from build123d import *

# Parameters (mm, degrees)
SKETCH_W      = 42
SKETCH_H      = 42
PAD_DEPTH     = 40
CHAMFER_SIZE  = 4
SKETCH001_W   = 44
SKETCH001_H   = 44
POCKET_DEPTH  = 32
PAD001_DEPTH  = 8
SKETCH003_R   = 11
SKETCH003_R_2 = 4.75
PAD002_DEPTH  = 2
PAD003_DEPTH  = 24.5
SKETCH005_R   = 1.7
HOLE_DEPTH    = 4.5
HOLE_TIPS_R   = 1.7


with BuildPart() as part:
    # Sketch → Pad (new body)
    with BuildSketch(Plane.XY):
        Rectangle(SKETCH_W, SKETCH_H)
    extrude(amount=PAD_DEPTH)

    # Chamfer
    chamfer_edges = [part.edges().sort_by_distance(p)[0] for p in [
        (21, -21, 20),
        (-21, -21, 20),
        (21, 21, 20),
        (-21, 21, 20),
    ]]
    chamfer(chamfer_edges, length=CHAMFER_SIZE)

    # Sketch001 (on Face5 of Chamfer) → Pocket (cut)
    with BuildSketch(Plane.XY.offset(40)):
        Rectangle(SKETCH001_W, SKETCH001_H)
        Polygon((-21, -12.868272), (-12.868272, -21), (12.868272, -21), (21, -12.868272), (21, 12.868272), (12.868272, 21), (-12.868272, 21), (-21, 12.868272), align=None, mode=Mode.SUBTRACT)
    extrude(amount=-POCKET_DEPTH, mode=Mode.SUBTRACT)

    # Sketch002 (on Face9 of Pocket) → Pad001 (join)
    with BuildSketch(Plane.XY.offset(40)):
        Polygon((-17, 21), (17, 21), (21, 17), (21, -17), (17, -21), (-17, -21), (-21, -17), (-21, 17), align=None)
    extrude(amount=-PAD001_DEPTH)

    # Sketch003 (on Face26 of Pad001) → Pad002 (join)
    with BuildSketch(Plane.XY.offset(40)):
        Circle(SKETCH003_R)
        Circle(SKETCH003_R_2, mode=Mode.SUBTRACT)
    extrude(amount=PAD002_DEPTH)

    # Sketch004 (on Face14 of Pad002) → Pad003 (join)
    with BuildSketch(Plane.XY.offset(40)):
        with BuildLine():
            ThreePointArc((-2, -1.5), (2.5, 0), (-2, 1.5))
            Line((-2, 1.5), (-2, -1.5))
        make_face()
    extrude(amount=PAD003_DEPTH)

    # Sketch005 (on Face14 of Pad003) → Hole (cut)
    with BuildSketch(Plane.XY.offset(40)):
        with Locations((-15.5, 15.5)):
            Circle(SKETCH005_R)
        with Locations((15.5, 15.5)):
            Circle(SKETCH005_R)
        with Locations((15.5, -15.5)):
            Circle(SKETCH005_R)
        with Locations((-15.5, -15.5)):
            Circle(SKETCH005_R)
    extrude(amount=-HOLE_DEPTH, mode=Mode.SUBTRACT)

    # Hole tips → Hole tip 1 section 0
    with BuildSketch(Plane.XY.offset(35.5), mode=Mode.PRIVATE) as hole_tip_1_s0:
        with Locations((-15.5, 15.5)):
            Circle(HOLE_TIPS_R)
    loft([hole_tip_1_s0.sketch, Vertex(-15.5, 15.5, 34.478537)], mode=Mode.SUBTRACT)

    # Hole tips → Hole tip 2 section 0
    with BuildSketch(Plane.XY.offset(35.5), mode=Mode.PRIVATE) as hole_tip_2_s0:
        with Locations((15.5, 15.5)):
            Circle(HOLE_TIPS_R)
    loft([hole_tip_2_s0.sketch, Vertex(15.5, 15.5, 34.478537)], mode=Mode.SUBTRACT)

    # Hole tips → Hole tip 3 section 0
    with BuildSketch(Plane.XY.offset(35.5), mode=Mode.PRIVATE) as hole_tip_3_s0:
        with Locations((15.5, -15.5)):
            Circle(HOLE_TIPS_R)
    loft([hole_tip_3_s0.sketch, Vertex(15.5, -15.5, 34.478537)], mode=Mode.SUBTRACT)

    # Hole tips → Hole tip 4 section 0
    with BuildSketch(Plane.XY.offset(35.5), mode=Mode.PRIVATE) as hole_tip_4_s0:
        with Locations((-15.5, -15.5)):
            Circle(HOLE_TIPS_R)
    loft([hole_tip_4_s0.sketch, Vertex(-15.5, -15.5, 34.478537)], mode=Mode.SUBTRACT)


solid = part.part
Check sheet for the modelled part. Datum: model origin and axes. Units: mm. A direction names the side the tool comes from. Coordinates: 2 decimals unless noted, no trailing zeros. Loops run counter-clockwise (first coordinate to the right, second up) from the corner with the lowest first, then second, coordinate; pieces in that order, holes last. Notation, with made-up numbers: (45, -20) -> (87, -20) arc R21 ccw to (87, 11) -> close; hole circle Ø4 at (-14, 81.25). An arc over 180 degrees is marked (long way). Answer in a Markdown table with one row per item.
1. Sectioned sample at D-D, the plane z = 19.5. Record the boundary of the cut face in (x, y).
Check values:
| item | result |
|---|---|
| outline | (-21, -12.87) -> (-12.87, -21) -> (12.87, -21) -> (21, -12.87) -> (21, 12.87) -> (12.87, 21) -> (-12.87, 21) -> (-21, 12.87) -> close |
2. Release check for a two-part mould opening along X. For faces 1 (the face through (17.07, -16.15, 37.78)), 2 (the face through (16.88, -16.99, 20.17)), 3 (the face through (-2.38, -10.74, 40.99)), 4 (the face through (-19, -19, 4)) record: released by +X, released by -X, zero draft, split by the parting line, or undercut.
Check values:
| item | result |
|---|---|
| face 1 | undercut |
| face 2 | released by +X |
| face 3 | split by the parting line |
| face 4 | released by -X |
3. Sectioned sample at C-C, the plane y = 0. Record the boundary of the cut face in (x, z).
Check values:
| item | result |
|---|---|
| outline | (-21, 0) -> (21, 0) -> (21, 40) -> (11, 40) -> (11, 42) -> (4.75, 42) -> (4.75, 40) -> (2.5, 40) -> (2.5, 64.5) -> (-2, 64.5) -> (-2, 40) -> (-4.75, 40) -> (-4.75, 42) -> (-11, 42) -> (-11, 40) -> (-21, 40) -> close |
4. Access from +Z, -Z, +X, -X, +Y, -Y to the whole of each face (thin tool, end or side, straight path). Record for faces 5 (the face through (-16.99, -16.88, 20.17)), 6 (the face through (21, 0, 20)), 7 (the face through (10, -9, 40)), 8 (the face through (18, 18, 32)), 9 (the face through (-18, 18, 8)).
Check values:
| item | result |
|---|---|
| face 5 | -X, -Y |
| face 6 | +Z, -Z, +X, +Y, -Y |
| face 7 | +Z |
| face 8 | +X, +Y |
| face 9 | -X, +Y |
5. Sectioned sample at A-A, the plane z = 41. Record the boundary of the cut face in (x, y).
Check values:
| item | result |
|---|---|
| outline | circle Ø22 at (0, 0); (-2, -1.5) arc R2.5 ccw (long way) to (-2, 1.5) -> close; hole circle Ø9.5 at (0, 0) |
6. Go/stop test with flat-tipped pins: pin 1 (12 mm diameter, centred on x = 5, y = -7, fed in from +Z); pin 2 (4 mm diameter, centred on x = -15.5, y = -15.5, fed in from +Z); pin 3 (2 mm diameter, centred on x = -15.5, z = 17, fed in from +Y). Record where each tip stops, or that it passes through.
Check values:
| item | result |
|---|---|
| pin 1 | stops at z = 42 |
| pin 2 | stops at z = 40 |
| pin 3 | stops at y = 19.37 |
7. Material ranges on line 1 along Y through (x, z) = (-15.5, 38.3); line 2 along Y through (x, z) = (0, 41.05); line 3 along X through (y, z) = (15, 37), recorded low to high. Write a range as [from, to].
Check values:
| item | result |
|---|---|
| line 1 | y = [-21, -17.2], [-13.8, 13.8], [17.2, 21] |
| line 2 | y = [-11, -4.75], [-2.5, 2.5], [4.75, 11] |
| line 3 | x = [-21, -17.12], [-13.88, 13.88], [17.12, 21] |
8. Sectioned sample at B-B, the plane x = 0. Record the boundary of the cut face in (y, z).
Check values:
| item | result |
|---|---|
| outline | (-21, 0) -> (21, 0) -> (21, 40) -> (11, 40) -> (11, 42) -> (4.75, 42) -> (4.75, 40) -> (2.5, 40) -> (2.5, 64.5) -> (-2.5, 64.5) -> (-2.5, 40) -> (-4.75, 40) -> (-4.75, 42) -> (-11, 42) -> (-11, 40) -> (-21, 40) -> close |
